from build123d import *

# Parameters (mm, degrees)
BOSS_EXTRUDE1_DEPTH   = 25
BOSS_EXTRUDE3_DEPTH   = 70
SKETCH7_R             = 36.833333333
BOSS_EXTRUDE4_DEPTH   = 121
SKETCH8_R             = 18.5
CUT_EXTRUDE2_DEPTH    = 232
SKETCH9_R             = 42.666666667
BOSS_EXTRUDE5_DEPTH   = 121
SKETCH10_R            = 18.5
CUT_EXTRUDE3_DEPTH    = 222
CHAMFER1_SIZE         = 2
CHAMFER1_SIZE2        = 1.154700538
CHAMFER1_PART_2_SIZE  = 2
CHAMFER1_PART_2_SIZE2 = 1.154700538
CHAMFER1_PART_3_SIZE  = 2
CHAMFER1_PART_3_SIZE2 = 1.154700538
CHAMFER1_PART_4_SIZE  = 2
CHAMFER1_PART_4_SIZE2 = 1.154700538
CUT_EXTRUDE4_DEPTH    = 20
CUT_EXTRUDE5_DEPTH    = 20
SKETCH16_R            = 36.833333333
SKETCH16_R_2          = 26.833333333
CUT_EXTRUDE7_DEPTH    = 30
BOSS_EXTRUDE7_REACH   = 114.667
SKETCH18_W            = 15
SKETCH18_H            = 30


with BuildPart() as part:
    # Sketch1 → Boss-Extrude1 (new body)
    with BuildSketch(Plane.XY):
        with BuildLine():
            Line((10, 0), (201, 0))
            ThreePointArc((201, 0), (208.071067812, 2.928932188), (211, 10))
            Line((211, 10), (211, 211))
            ThreePointArc((211, 211), (208.071067812, 218.071067812), (201, 221))
            Line((201, 221), (10, 221))
            ThreePointArc((10, 221), (2.928932188, 218.071067812), (0, 211))
            Line((0, 211), (0, 10))
            ThreePointArc((0, 10), (2.928932188, 2.928932188), (10, 0))
        make_face()
    extrude(amount=BOSS_EXTRUDE1_DEPTH)

    # Sketch5 → Boss-Extrude3 (add)
    with BuildSketch(Plane.XY.offset(25)):
        with BuildLine():
            Line((46, 0), (46, 80))
            ThreePointArc((46, 80), (106.104076401, 104.895923599), (131, 165))
            Line((131, 165), (211, 165))
            Line((211, 165), (211, 150))
            Line((211, 150), (144.868599666, 150))
            ThreePointArc((144.868599666, 150), (116.710678119, 94.289321881), (61, 66.131400334))
            Line((61, 66.131400334), (61, 0))
            Line((61, 0), (46, 0))
        make_face()
    extrude(amount=BOSS_EXTRUDE3_DEPTH)

    # Sketch7 → Boss-Extrude4 (add)
    with BuildSketch(Plane(origin=(0, -10, 0), x_dir=(-1, 0, 0), z_dir=(0, -1, 0))):
        with Locations((-53.5, -95)):
            Circle(SKETCH7_R)
    extrude(amount=-BOSS_EXTRUDE4_DEPTH)

    # Sketch8 → Cut-Extrude2 (cut, through all)
    with BuildSketch(Plane.XZ.offset(10)):
        with Locations((53.5, 95)):
            Circle(SKETCH8_R)
    extrude(amount=-CUT_EXTRUDE2_DEPTH, mode=Mode.SUBTRACT)

    # Sketch9 → Boss-Extrude5 (add)
    with BuildSketch(Plane(origin=(221, 0, 0), x_dir=(0, 0, -1), z_dir=(1, 0, 0))):
        with Locations((-95, 157.5)):
            Circle(SKETCH9_R)
    extrude(amount=-BOSS_EXTRUDE5_DEPTH)

    # Sketch10 → Cut-Extrude3 (cut, through all)
    with BuildSketch(Plane(origin=(221, 0, 0), x_dir=(0, 0, -1), z_dir=(1, 0, 0))):
        with Locations((-95, 157.5)):
            Circle(SKETCH10_R)
    extrude(amount=-CUT_EXTRUDE3_DEPTH, mode=Mode.SUBTRACT)

    # Chamfer1
    chamfer1_edges = [part.edges().sort_by_distance(p)[0] for p in [
        (35, 111, 95),
    ]]
    chamfer1_side = [part.faces().sort_by_distance(p)[0] for p in [
        (35, 50.5, 95),
    ]]
    chamfer(chamfer1_edges, length=CHAMFER1_SIZE, length2=CHAMFER1_SIZE2, reference=chamfer1_side[0])

    # Chamfer1 part 2
    chamfer1_part_2_edges = [part.edges().sort_by_distance(p)[0] for p in [
        (35, -10, 95),
    ]]
    chamfer1_part_2_side = [part.faces().sort_by_distance(p)[0] for p in [
        (89.291529342, -10, 95),
    ]]
    chamfer(chamfer1_part_2_edges, length=CHAMFER1_PART_2_SIZE, length2=CHAMFER1_PART_2_SIZE2, reference=chamfer1_part_2_side[0])

    # Chamfer1 part 3
    chamfer1_part_3_edges = [part.edges().sort_by_distance(p)[0] for p in [
        (100, 157.5, 113.5),
    ]]
    chamfer1_part_3_side = [part.faces().sort_by_distance(p)[0] for p in [
        (160.5, 157.5, 113.5),
    ]]
    chamfer(chamfer1_part_3_edges, length=CHAMFER1_PART_3_SIZE, length2=CHAMFER1_PART_3_SIZE2, reference=chamfer1_part_3_side[0])

    # Chamfer1 part 4
    chamfer1_part_4_edges = [part.edges().sort_by_distance(p)[0] for p in [
        (221, 157.5, 113.5),
    ]]
    chamfer1_part_4_side = [part.faces().sort_by_distance(p)[0] for p in [
        (221, 157.5, 136.459871093),
    ]]
    chamfer(chamfer1_part_4_edges, length=CHAMFER1_PART_4_SIZE, length2=CHAMFER1_PART_4_SIZE2, reference=chamfer1_part_4_side[0])

    # Sketch11 → Cut-Extrude4 (cut)
    with BuildSketch(Plane.XY.offset(25)):
        with BuildLine():
            Line((192, 141), (160.039466852, 141))
            ThreePointArc((160.039466852, 141), (154.063323806, 139.017837257), (150.456318377, 133.857142857))
            ThreePointArc((150.456318377, 133.857142857), (123.074639149, 87.925360851), (77.142857143, 60.543681623))
            ThreePointArc((77.142857143, 60.543681623), (71.982162743, 56.936676194), (70, 50.960533148))
            Line((70, 50.960533148), (70, 19))
            ThreePointArc((70, 19), (72.92893248, 11.928931897), (80.000000825, 9))
            Line((80.000000825, 9), (192.000000825, 9.000009238))
            ThreePointArc((192.000000825, 9.000009238), (199.071068103, 11.928941718), (202, 19.000009238))
            Line((202, 19.000009238), (202, 131))
            ThreePointArc((202, 131), (199.071067812, 138.071067812), (192, 141))
        make_face()
    extrude(amount=-CUT_EXTRUDE4_DEPTH, mode=Mode.SUBTRACT)

    # Sketch12 → Cut-Extrude5 (cut)
    with BuildSketch(Plane.XY.offset(25)):
        with BuildLine():
            Line((19, 212), (112, 212))
            ThreePointArc((112, 212), (119.071067812, 209.071067812), (122, 202))
            Line((122, 202), (122, 165))
            ThreePointArc((122, 165), (99.74011537, 111.25988463), (46, 89))
            Line((46, 89), (19, 89))
            ThreePointArc((19, 89), (11.928932188, 91.928932188), (9, 99))
            Line((9, 99), (9, 202))
            ThreePointArc((9, 202), (11.928932188, 209.071067812), (19, 212))
        make_face()
    extrude(amount=-CUT_EXTRUDE5_DEPTH, mode=Mode.SUBTRACT)

    # Sketch16 → Cut-Extrude7 (cut)
    with BuildSketch(Plane(origin=(0, 20, 0), x_dir=(-1, 0, 0), z_dir=(0, -1, 0))):
        with Locations((-53.5, -95)):
            Circle(SKETCH16_R)
        with Locations((-53.5, -95)):
            Circle(SKETCH16_R_2, mode=Mode.SUBTRACT)
    extrude(amount=-CUT_EXTRUDE7_DEPTH, mode=Mode.SUBTRACT)

    # Sketch18 → Boss-Extrude7 (add, up to next)
    with BuildSketch(Plane.XY.offset(25), mode=Mode.PRIVATE) as boss_extrude7_sk1:
        with Locations((53.5, 35)):
            Rectangle(SKETCH18_W, SKETCH18_H)
    boss_extrude7_tool1 = extrude(boss_extrude7_sk1.sketch, amount=BOSS_EXTRUDE7_REACH, mode=Mode.PRIVATE) - part.part
    add(boss_extrude7_tool1.solids().sort_by_distance((53.5, 35, 25))[0])


solid = part.part
For this review, take the finished solid that the model builds, in its own axes (mm). A direction names the side the tool comes from. Round coordinates to 2 decimals unless told otherwise and drop trailing zeros. Loops run counter-clockwise (first coordinate to the right, second up) from the corner with the lowest first, then second, coordinate; pieces in that order, holes last. Notation, with made-up numbers: (0, 44.25) - (43, 44.25) arc R26 ccw to (43, 63.25) - close; hole circle Ø7 at (73, 74.5). An arc over 180 degrees is marked (long way). Answer as CSV lines item,"result".
(1) Consider section B-B on y = 157.5. Give the boundary of the cut face in (x, z).
Checked values:
outline,"(0, 0) - (211, 0) - (211, 52.33) - (221, 52.33) - (221, 74.5) - (219.85, 76.5) - (102, 76.5) - (100, 75.35) - (100, 52.33) - (130.67, 52.33) - (130.67, 25) - (121.63, 25) - (121.63, 5) - (9, 5) - (9, 25) - (0, 25) - close; (100, 114.65) - (102, 113.5) - (219.85, 113.5) - (221, 115.5) - (221, 137.67) - (100, 137.67) - close"
(2) Consider section A-A on x = 168.5. Give the boundary of the cut face in (y, z).
Checked values:
outline,"(0, 0) - (221, 0) - (221, 25) - (165, 25) - (165, 53) arc R42.67 ccw (long way) to (150, 53) - (150, 25) - (141, 25) - (141, 5) - (9, 5) - (9, 25) - (0, 25) - close; hole circle Ø37 at (157.5, 95)"
(3) Wall thickness on line 1 (Y direction, x = 172, z = 95); line 2 (Z direction, x = 53.5, y = 39); line 3 (Z direction, x = 60, y = 108.5): over which ranges is each line inside the solid? List them lowest first.
Checked values:
line 1,"y = 114.83 to 139, 176 to 200.17"
line 2,"z = 0 to 76.5, 113.5 to 121.83"
line 3,"z = 0 to 5, 58.74 to 77.68, 112.32 to 131.26"
(4) Tool access review of faces 1 (the face through (178, 150, 39)), 2 (the face through (54.57, 34.79, 121.81)), 3 (the face through (105, 111, 25)): name each direction out of +Z, -Z, +X, -X, +Y, -Y from which nothing blocks a thin tool from reaching the whole face with its end or side.
Checked values:
face 1,"+X, -Y"
face 2,"none"
face 3,"-X, +Y"
(5) Insertion check: P1, Ø3, axis at y = 39.5, z = 51.5, coming from the -X side; P2, Ø22, axis at y = 17.5, z = 45, coming from the +X side; P3, Ø22, axis at y = 126, z = 17.5, coming from the +X side; P4, Ø22.5, axis at x = 173.5, z = 32, coming from the +Y side. Each pin has a flat end and moves straight along its axis. Give the tip position at first contact, or say it passes through.
Checked values:
P1,"stops at x = 46"
P2,"stops at x = 61"
P3,"stops at x = 211"
P4,"stops at y = 221"
(6) Consider section C-C on x = 53.5. Give the boundary of the cut face in (y, z).
Checked values:
outline,"(-10, 58.17) - (0, 58.17) - (0, 0) - (221, 0) - (221, 25) - (212, 25) - (212, 5) - (89.37, 5) - (89.37, 25) - (80.33, 25) - (80.33, 58.17) - (111, 58.17) - (111, 75.35) - (109, 76.5) - (-8.85, 76.5) - (-10, 74.5) - close; (-10, 115.5) - (-8.85, 113.5) - (109, 113.5) - (111, 114.65) - (111, 131.83) - (50, 131.83) - (50, 121.83) - (20, 121.83) - (20, 131.83) - (-10, 131.83) - close"
(7) Mouldability with a two-part tool opening along Z and no side actions: class faces 4 (the face through (36.504, 4.79, 127.678)), 5 (the face through (211, 109, 14)) as +Z half, -Z half, draft (parallel to the pull), parting line (faces both ways), or undercut.
Checked values:
face 4,"undercut"
face 5,"draft"
